```python
from build123d import *

# Parameters (mm, degrees)
SKETCH1_W           = 1
SKETCH1_H           = 10
BOSS_EXTRUDE1_DEPTH = 45


with BuildPart() as part:
    # Sketch1 → Boss-Extrude1 (new body)
    with BuildSketch(Plane(origin=(0, 0, 0), x_dir=(-1, 0, 0), z_dir=(0, 1, 0))):
        with Locations((0.5, 7)):
            Rectangle(SKETCH1_W, SKETCH1_H)
        Polygon((1, 2), (0, 2), (0, 0), (31, 0), (31, 2), (30, 2), (29, 2), (28, 2), (27, 2), (26, 2), (25, 2), (24, 2), (23, 2), (22, 2), (21, 2), (20, 2), (19, 2), (18, 2), (17, 2), (16, 2), (15, 2), (14, 2), (13, 2), (12, 2), (11, 2), (10, 2), (9, 2), (8, 2), (7, 2), (6, 2), (5, 2), (4, 2), (3, 2), (2, 2), align=None)
        with Locations((2.5, 7)):
            Rectangle(SKETCH1_W, SKETCH1_H)
        with Locations((4.5, 7)):
            Rectangle(SKETCH1_W, SKETCH1_H)
        with Locations((6.5, 7)):
            Rectangle(SKETCH1_W, SKETCH1_H)
        with Locations((8.5, 7)):
            Rectangle(SKETCH1_W, SKETCH1_H)
        with Locations((10.5, 7)):
            Rectangle(SKETCH1_W, SKETCH1_H)
        with Locations((12.5, 7)):
            Rectangle(SKETCH1_W, SKETCH1_H)
        with Locations((14.5, 7)):
            Rectangle(SKETCH1_W, SKETCH1_H)
        with Locations((16.5, 7)):
            Rectangle(SKETCH1_W, SKETCH1_H)
        with Locations((18.5, 7)):
            Rectangle(SKETCH1_W, SKETCH1_H)
        with Locations((20.5, 7)):
            Rectangle(SKETCH1_W, SKETCH1_H)
        with Locations((22.5, 7)):
            Rectangle(SKETCH1_W, SKETCH1_H)
        with Locations((24.5, 7)):
            Rectangle(SKETCH1_W, SKETCH1_H)
        with Locations((26.5, 7)):
            Rectangle(SKETCH1_W, SKETCH1_H)
        with Locations((28.5, 7)):
            Rectangle(SKETCH1_W, SKETCH1_H)
        with Locations((30.5, 7)):
            Rectangle(SKETCH1_W, SKETCH1_H)
    extrude(amount=BOSS_EXTRUDE1_DEPTH)


solid = part.part
```
Here's how the part is built. I have some questions about the finished solid (model axes, mm). A direction names the side the tool comes from. Give positions to 0.01 mm unless a question says otherwise; leave off trailing zeros. Loops run counter-clockwise (first coordinate to the right, second up) from the corner with the lowest first, then second, coordinate; pieces in that order, holes last. Notation, with made-up numbers: M 75.25,70.5 L 100.25,70.5 A12 cw 100.25,82.5 Z; hole C 15.25,-14.75 d9. An arc over 180 degrees is marked long. Put each result on its own line as item: value. Start each with the question number.
(1) I want a section at A-A on z = 11.25. State how many separate pieces and enclosed holes the cut face has, then the cut area to 3 significant figures.
(2) I need wall thicknesses on line 1 along Z through (x, y) = (-9.5, 31.5). Which ranges of the line are inside material? Lowest first, please. Write a range as [from, to].
(3) Will this pin go through, and if not, where does the flat tip stop? pin 1 Ø0.8 at (x, y) = (-29.5, 18) entering from +Z.
(4) If we mould it in two halves opening along X, with no side actions, what happens to faces 1 (the flat face through (-9.5, 22.2, 2)), 2 (the flat face through (-26, 22, 7)), 3 (the flat face through (-6.5, 22.2, 12))? For each: +X half, -X half, draft (parallel to the pull), parting line (faces both ways), or undercut.
(5) For faces 4 (the flat face through (-5.5, 22.2, 2)), 5 (the flat face through (-24.5, 22.2, 12)), which set-ups out of +Z, -Z, +X, -X, +Y, -Y let a thin tool reach every point of the face, with its end or its side?
(6) I want a section at B-B on x = -23.5. Please give me the cut outline in (y, z).
Answer block:
1. separate pieces: 16
1. enclosed holes: 0
1. area: 720 mm^2
2. line 1: [0, 2]
3. pin 1: z = 2
4. face 1: undercut
4. face 2: undercut
4. face 3: draft
5. face 4: +Z, +Y, -Y
5. face 5: +Z, +X, -X, +Y, -Y
6. outline: M 0,0 L 45,0 L 45,2 L 0,2 Z
